```python
from build123d import *

# Parameters (mm, degrees)
F0_R     = 44.45
F0_R_2   = 31.242
F1_DEPTH = 2.54
F2_R     = 38.1
F2_R_2   = 31.242
F3_DEPTH = 5.08
F5_DEPTH = 2.54
F6_R     = 38.1
F6_R_2   = 31.242
F7_DEPTH = 2.54
F9_DEPTH = 2.54
F10_SIZE = 2.53999


# Not quite as in the source:
# - a fillet or chamfer is up to 0.001 mm smaller than in the source, because OpenCascade refuses the exact size


with BuildPart() as f1:
    # F0 (on Top) → F1 (new body)
    with BuildSketch(Plane.XY):
        Circle(F0_R)
        Circle(F0_R_2, mode=Mode.SUBTRACT)
    extrude(amount=F1_DEPTH)

    # F2 (on face) → F3 (join)
    with BuildSketch(Plane.XY.offset(2.54)):
        Circle(F2_R)
        Circle(F2_R_2, mode=Mode.SUBTRACT)
    extrude(amount=F3_DEPTH)

    # F4 (on face) → F5 (cut)
    with BuildSketch(Plane.XY.offset(7.62)):
        with BuildLine():
            ThreePointArc((-25.5919481677, -17.9196750245), (-27.0835882302, -15.5737539654), (-28.3607839843, -13.1045219598))
            Line((-28.3607839843, -13.1045219598), (-32.2805671366, -14.9157160518))
            ThreePointArc((-32.2805671366, -14.9157160518), (-31.5707150955, -16.3647043469), (-30.7958633586, -17.78))
            ThreePointArc((-30.7958633586, -17.78), (-26.0009342584, -24.2582979142), (-19.8703037457, -29.4904158847))
            Line((-19.8703037457, -29.4904158847), (-13.2034397333, -28.3148678826))
            ThreePointArc((-13.2034397333, -28.3148678826), (-20.0819705018, -23.9327604919), (-25.5919481677, -17.9196750245))
        make_face()
        with BuildLine():
            ThreePointArc((-17.9196750245, 25.5919481677), (-10.6853933178, 29.3578768586), (-2.7229197149, 31.1231147578))
            ThreePointArc((-2.7229197149, 31.1231147578), (0.0545275488, 31.2419524157), (2.8315430705, 31.1134203816))
            Line((2.8315430705, 31.1134203816), (3.2228945518, 35.4136492148))
            ThreePointArc((3.2228945518, 35.4136492148), (1.6131078579, 35.5233934618), (0, 35.56))
            ThreePointArc((0, 35.56), (-8.007835117, 34.646618547), (-15.6042974515, 31.9533957671))
            Line((-15.6042974515, 31.9533957671), (-17.9196750245, 25.5919481677))
        make_face()
        with BuildLine():
            Line((35.4746011972, -2.4629798824), (31.1231147578, 2.7229197149))
            ThreePointArc((31.1231147578, 2.7229197149), (31.2122645387, 1.3627569001), (31.242, 0))
            ThreePointArc((31.242, 0), (29.7795828432, -9.4466401268), (25.5292409138, -18.0088984218))
            Line((25.5292409138, -18.0088984218), (29.0576725848, -20.497933163))
            ThreePointArc((29.0576725848, -20.497933163), (29.9576072376, -19.1586891148), (30.7958633586, -17.78))
            ThreePointArc((30.7958633586, -17.78), (34.0087693754, -10.3883206328), (35.4746011972, -2.4629798824))
        make_face()
    extrude(amount=-F5_DEPTH, mode=Mode.SUBTRACT)

    # F6 (on face) → F7 (join)
    with BuildSketch(Plane.XY.offset(7.62)):
        Circle(F6_R)
        Circle(F6_R_2, mode=Mode.SUBTRACT)
    extrude(amount=F7_DEPTH)

    # F8 (on face) → F9 (cut)
    with BuildSketch(Plane.XY.offset(10.16)):
        with BuildLine():
            ThreePointArc((-25.5919481677, -17.9196750245), (-27.0835882302, -15.5737539654), (-28.3607839843, -13.1045219598))
            Line((-28.3607839843, -13.1045219598), (-32.2805671366, -14.9157160518))
            ThreePointArc((-32.2805671366, -14.9157160518), (-31.5707150955, -16.3647043469), (-30.7958633586, -17.78))
            Line((-30.7958633586, -17.78), (-25.5919481677, -17.9196750245))
        make_face()
        with BuildLine():
            ThreePointArc((28.3148678826, -13.2034397333), (27.0290606814, -15.6681984503), (25.5292409138, -18.0088984218))
            Line((25.5292409138, -18.0088984218), (29.0576725848, -20.497933163))
            ThreePointArc((29.0576725848, -20.497933163), (29.9576072376, -19.1586891148), (30.7958633586, -17.78))
            Line((30.7958633586, -17.78), (28.3148678826, -13.2034397333))
        make_face()
        with BuildLine():
            Line((0, 35.56), (-2.7229197149, 31.1231147578))
            ThreePointArc((-2.7229197149, 31.1231147578), (0.0545275488, 31.2419524157), (2.8315430705, 31.1134203816))
            Line((2.8315430705, 31.1134203816), (3.2228945518, 35.4136492148))
            ThreePointArc((3.2228945518, 35.4136492148), (1.6131078579, 35.5233934618), (0, 35.56))
        make_face()
    extrude(amount=-F9_DEPTH, mode=Mode.SUBTRACT)

    # F10 (size 2.54 in the source; OpenCascade refuses exactly that, so slightly less here)
    f10_edges = [f1.edges().sort_by_distance(p)[0] for p in [
        (-44.45, 0, 2.54),
    ]]
    chamfer(f10_edges, length=F10_SIZE)


solid = f1.part
```
The listing builds one solid part. Answer for the finished solid, in the listing's coordinates (mm). A direction names the side the tool comes from. Coordinates: 2 decimals unless noted, no trailing zeros. Loops run counter-clockwise (first coordinate to the right, second up) from the corner with the lowest first, then second, coordinate; pieces in that order, holes last. Notation, with made-up numbers: M 52.5,81 L 109.5,81 A17 cw 109.5,106 Z; hole C 30.5,29 d1. An arc over 180 degrees is marked long. Answer as CSV lines item,"result". Start each with the question number.
(1) Find the intervals of material crossed by L1, parallel to Y at x = 0, z = 3.5; L2, parallel to Z at x = 5.5, y = -39; L3, parallel to X at y = 2, z = 0.75, in increasing order. Write a range as [from, to].
(2) For faces 1 (the flat face through (-30.3, -9.3, 0)), 2 (the flat face through (27.269, -19.236, 7.656)), 3 (the flat face through (32, -7, 7.62)), determine the directions among +Z, -Z, +X, -X, +Y, -Y from which every point of the face is accessible in a straight line to the end or side of a thin tool.
(3) The mould has two halves that part along X. Classify faces 4 (the flat face through (-1.342, 33.373, 8.908)), 5 (the cylindrical face through (-30.235, -23.183, 6.297)), 6 (the flat face through (5, -31, 10.16)): pulls with the +X half, pulls with the -X half, needs draft (parallel to the pull), parting line crosses it, or undercut.
(4) The part is cut by section A-A (z = 4). Give the vertices of the cut face in (x, y).
(5) Given pin 1 (1.5 mm diameter, centred on y = 23, z = 4, fed in from +X); pin 2 (3 mm diameter, centred on y = 21.5, z = 7, fed in from -X); pin 3 (1 mm diameter, centred on x = -17.5, y = -35.5, fed in from +Z); pin 4 (5 mm diameter, centred on x = -8.5, y = 26, fed in from -Z), each flat-ended and moving along its own axis, determine where each tip first touches the part or whether it passes through.
Determined:
1,L1,"[-38.1, -31.24], [31.24, 38.1]"
1,L2,"[0, 2.54]"
1,L3,"[-43.65, -31.18], [31.18, 43.65]"
2,face 1,"-Z, +X, -X, +Y, -Y"
2,face 2,"+Z"
2,face 3,"none"
3,face 4,"undercut"
3,face 5,"parting line crosses it"
3,face 6,"needs draft"
4,outline,"C 0,0 d76.2; hole C 0,0 d62.48"
5,pin 1,"x = 30.93"
5,pin 2,"x = -32.43"
5,pin 3,"z = 2.54"
5,pin 4,"through"
